For this review, take the finished solid that the model builds, in its own axes (mm). Give positions to 0.01 mm unless a question says otherwise; leave off trailing zeros. Loops run counter-clockwise (first coordinate to the right, second up) from the corner with the lowest first, then second, coordinate; pieces in that order, holes last.
```python
from build123d import *

# Parameters (mm, degrees)
F0_W     = 304.8
F0_H     = 177.8
F1_DEPTH = 25.4
F2_R     = 19.05
F3_R     = 6.35


with BuildPart() as f1:
    # F0 (on Front) → F1 (new body, symmetric)
    with BuildSketch(Plane.XZ):
        with Locations((152.4, 88.9)):
            Rectangle(F0_W, F0_H)
    extrude(amount=F1_DEPTH, both=True)

    # F2
    f2_edges = [f1.edges().sort_by_distance(p)[0] for p in [
        (304.8, -25.4, 88.9),
        (304.8, 25.4, 88.9),
        (0, 25.4, 88.9),
        (0, -25.4, 88.9),
    ]]
    fillet(f2_edges, radius=F2_R)

    # F3
    f3_edges = [f1.edges().sort_by_distance(p)[0] for p in [
        (152.4, -25.4, 177.8),
        (152.4, -25.4, 0),
    ]]
    fillet(f3_edges, radius=F3_R)


solid = f1.part
```
Q1. Consider section A-A on z = 161. Give the boundary of the cut face in (x, y).
Answers:
outline: (0, -6.35) arc R19.05 ccw to (19.05, -25.4) - (285.75, -25.4) arc R19.05 ccw to (304.8, -6.35) - (304.8, 6.35) arc R19.05 ccw to (285.75, 25.4) - (19.05, 25.4) arc R19.05 ccw to (0, 6.35) - close
Q2. For pin 1 Ø1 at (y, z) = (-14, 72.5) entering from -X; pin 2 Ø8 at (y, z) = (-9.5, 44) entering from -X; pin 3 Ø2 at (y, z) = (-16.5, 20) entering from -X, all flat-tipped, find the tip position at first contact; note any pin that passes through.
Answers:
pin 1: stops at x = 1.39
pin 2: stops at x = 0
pin 3: stops at x = 2.34
Q3. For probe 1 along X at (y, z) = (8, 136.5); probe 2 along X at (y, z) = (-7.5, 81), list the stretches that pass through material, from the lowest coordinate up.
Answers:
probe 1: x = 0.07 to 304.73
probe 2: x = 0.03 to 304.77
Q4. Mouldability with a two-part tool opening along X and no side actions: class faces 1 (the cylindrical face through (302.89, 0.09, 1.81)), 2 (the cylindrical face through (1.91, -0.09, 175.99)), 3 (the flat face through (151, 25.4, 90)) as +X half, -X half, draft (parallel to the pull), parting line (faces both ways), or undercut.
Answers:
face 1: +X half
face 2: -X half
face 3: draft
